Source: CAD feature listing. Evaluate the final solid. Frame: model axes, mm. Round coordinates to 2 decimals unless told otherwise and drop trailing zeros. Loops run counter-clockwise (first coordinate to the right, second up) from the corner with the lowest first, then second, coordinate; pieces in that order, holes last. Notation, with made-up numbers: (-6.5, 55) -> (51.5, 55) arc R14 cw to (51.5, 67) -> close; hole circle Ø7 at (33, -14). An arc over 180 degrees is marked (long way). Return JSON: item names as keys, results as strings. Group by question number.
```python
from build123d import *

# Parameters (mm, degrees)
BOSS_EXTRUDE1_START = -21
SKETCH2_R           = 10.322343774
SKETCH2_R_2         = 9.5
BOSS_EXTRUDE1_DEPTH = 21
FILLET1_R           = 0.5


with BuildPart() as part:
    # Sketch1 → Revolve1 (revolve)
    with BuildSketch(Plane.XY, mode=Mode.PRIVATE) as revolve1_sk:
        with BuildLine():
            Line((6, 11.335), (-14.512496096, 10.822187598))
            ThreePointArc((-14.512496096, 10.822187598), (-14.857944163, 10.671451174), (-15, 10.322343774))
            Line((-15, 10.322343774), (6, 10.322343774))
            Line((6, 10.322343774), (6, 11.335))
        make_face()
    revolve(revolve1_sk.sketch.rotate(Axis((-15.624243475, 0, 0), (1, 0, 0)), 90), axis=Axis((-15.624243475, 0, 0), (1, 0, 0)))

    # Sketch2 → Boss-Extrude1 (add)
    with BuildSketch(Plane(origin=(6, 0, 0), x_dir=(0, 0, -1), z_dir=(1, 0, 0)).offset(BOSS_EXTRUDE1_START)):
        Circle(SKETCH2_R)
        Circle(SKETCH2_R_2, mode=Mode.SUBTRACT)
    extrude(amount=BOSS_EXTRUDE1_DEPTH)

    # Fillet1
    fillet1_edges = [part.edges().sort_by_distance(p)[0] for p in [
        (-15, 0, 9.5),
    ]]
    fillet(fillet1_edges, radius=FILLET1_R)


solid = part.part
```
(1) Mould query, pull axis Z, two halves, no side actions, for faces 1 (the face through (-4.4, -3.327, 10.564)), 2 (the face through (6, -8, 6)), 3 (the face through (-4.39, -8.43, -4.38)). Classes: released by +Z, released by -Z, zero draft, split by the parting line, or undercut.
(2) Cut plane C-C (x = -4). Return loops of the section in (y, z) (3 decimals).
(3) Pin query (flat end, axial travel): pin 1 (1 mm diameter, centred on x = -1.5, y = 7, fed in from -Z); pin 2 (10 mm diameter, centred on x = -2, z = -7, fed in from -Y); pin 3 (6 mm diameter, centred on x = -4.5, z = -6.5, fed in from -Y); pin 4 (8 mm diameter, centred on x = 3.5, y = -1, fed in from -Z) (3 decimals). Return the tip coordinate at first contact, or that it passes through.
(4) Cut plane B-B (x = -7.5). Return loops of the section in (y, z) (1 decimal).
(5) Ray query, line 1 (Y direction, x = 1, z = 0); line 2 (Y direction, x = 0.5, z = 7.75); line 3 (Z direction, x = 2, y = -8.5). Return the intervals inside material, ascending.
Answers follow:
{
 "1": {"face 1": "split by the parting line", "face 2": "zero draft", "face 3": "undercut"},
 "2": {"outline": "circle Ø22.17 at (0, 0); hole circle Ø19 at (0, 0)"},
 "3": {"pin 1": "z = -9.06", "pin 2": "y = -10.96", "pin 3": "y = -10.51", "pin 4": "z = -11.335"},
 "4": {"outline": "circle Ø22 at (0, 0); hole circle Ø19 at (0, 0)"},
 "5": {"line 1": "-11.21 to -9.5, 9.5 to 11.21", "line 2": "-8.08 to -5.49, 5.49 to 8.08", "line 3": "-7.35 to -4.24, 4.24 to 7.35"}
}
